from build123d import *

# Parameters (mm, degrees)
SKETCH1_R           = 2.75
BOSS_EXTRUDE1_DEPTH = 8
SKETCH5_R           = 2.25
BOSS_EXTRUDE2_DEPTH = 19
SKETCH6_R           = 6
BOSS_EXTRUDE4_DEPTH = 1.5
CUT_EXTRUDE1_DEPTH  = 1.5
CIRPATTERN1_COUNT   = 4
SKETCH11_R          = 1.4
BOSS_EXTRUDE5_DEPTH = 3
SKETCH12_R          = 2.2
BOSS_EXTRUDE6_DEPTH = 2.5


with BuildPart() as part:
    # Sketch1 → Boss-Extrude1 (new body)
    with BuildSketch(Plane.XY):
        with Locations((0, -0.147315355)):
            Circle(SKETCH1_R)
    extrude(amount=BOSS_EXTRUDE1_DEPTH)

    # Sketch4 → Revolve2 (revolve)
    with BuildSketch(Plane(origin=(0, 0, 0), x_dir=(1, 0, 0), z_dir=(0, 1, 0)), mode=Mode.PRIVATE) as revolve2_sk:
        Polygon((0, 0), (0, 2), (-2, 0), align=None)
    revolve(revolve2_sk.sketch.rotate(Axis((0, 0, 0), (0, 0, -1)), 180), axis=Axis((0, 0, 0), (0, 0, -1)))

    # Sketch5 → Boss-Extrude2 (add)
    with BuildSketch(Plane.XY.offset(8)):
        Circle(SKETCH5_R)
    extrude(amount=BOSS_EXTRUDE2_DEPTH)

    # Sketch6 → Boss-Extrude4 (add)
    with BuildSketch(Plane.XY.offset(8)):
        Circle(SKETCH6_R)
    extrude(amount=BOSS_EXTRUDE4_DEPTH)

    # Sketch7 → Cut-Extrude1 (cut)
    with BuildSketch(Plane(origin=(0, 0, 8), x_dir=(-1, 0, 0), z_dir=(0, 0, -1))):
        with BuildLine():
            ThreePointArc((0.5, -4.974937186), (3.535533906, -3.535533906), (4.974937186, -0.5))
            Line((4.974937186, -0.5), (2.727290513, -0.5))
            ThreePointArc((2.727290513, -0.5), (1.996550566, -2.038422395), (0.5, -2.851478812))
            Line((0.5, -2.851478812), (0.5, -4.974937186))
        make_face()
    cut_extrude1 = extrude(amount=-CUT_EXTRUDE1_DEPTH, mode=Mode.SUBTRACT)

    # CirPattern1: Cut-Extrude1 ×4 about axis
    cirpattern1_axis = Axis((0, 0, 0), (0, 0, 1))
    for i in range(1, CIRPATTERN1_COUNT):
        add(cut_extrude1.rotate(cirpattern1_axis, i * 360 / CIRPATTERN1_COUNT), mode=Mode.SUBTRACT)

    # Sketch10 → Revolve3 (revolve)
    with BuildSketch(Plane(origin=(0, 0, 0), x_dir=(0, 0, -1), z_dir=(1, 0, 0))):
        with BuildLine():
            Line((-27, 0), (-29, 0))
            Line((-29, 0), (-29, 1.4))
            add(Edge.make_bspline(
                [(-29, 1.4), (-28.086565691, 2.25), (-27, 2.25)],
                knots=[0, 0, 0, 1, 1, 1], degree=2))
            Line((-27, 2.25), (-27, 0))
        make_face()
    revolve(axis=Axis((0, 0, 27), (0, 0, 1)))

    # Sketch11 → Boss-Extrude5 (add)
    with BuildSketch(Plane.XY.offset(29)):
        Circle(SKETCH11_R)
    extrude(amount=BOSS_EXTRUDE5_DEPTH)

    # Sketch12 → Boss-Extrude6 (add)
    with BuildSketch(Plane.XY.offset(32)):
        Circle(SKETCH12_R)
    extrude(amount=BOSS_EXTRUDE6_DEPTH)


solid = part.part
Read the model definition and answer for the solid it produces. Units are mm, in the model's axes. A direction names the side the tool comes from. Give positions to 0.01 mm unless a question says otherwise; leave off trailing zeros. Write each loop counter-clockwise with the first axis right and the second up, starting at its lowest first coordinate (ties: lowest second). Pieces come first, ordered by that corner, then holes. Notation, with made-up numbers: (20.25, 1.5) - (34.25, 1.5) arc R33 ccw to (34.25, 33.5) - close; hole circle Ø11 at (15.5, 0.5). An arc over 180 degrees is marked (long way). Answer in a Markdown table with one row per item. Add a question column.
Item 1: Determine the mould class of faces 5 (the face through (0, 1, -1)), 6 (the face through (-0.5, -4, 9)), 7 (the face through (0, 3, 8)) for opening direction X: pulls with the +X half, pulls with the -X half, needs draft (parallel to the pull), parting line crosses it, or undercut.
Item 2: Section B-B, the plane z = 16 is taken. Write down the section's boundary in (x, y), and give its area (3 significant figures).
Item 3: Flat-ended cylindrical pins translate along their axes: P1, Ø1.6, axis at x = -4, z = 8.5, coming from the +Y side; P2, Ø1, axis at x = 0.5, y = -2.5, coming from the -Z side; P3, Ø0.8, axis at y = 4.5, z = 8.5, coming from the +X side; P4, Ø1, axis at x = 3, z = 28, coming from the +Y side. Find the tip coordinate at first contact, or state that the pin passes through.
Item 4: Section A-A, the plane x = -4 is taken. Write down the section's boundary in (y, z).
Item 5: Section C-C, the plane y = 1 is taken. Count the separate pieces of the cut face and the enclosed holes in it, and give its area (3 significant figures).
Item 6: A tool of negligible diameter and unlimited length cuts with its end or side. For faces 1 (the face through (-0.5, 4, 9)), 2 (the face through (1, -2, 0)), 3 (the face through (2.021, -2.013, 8.74)), 4 (the face through (0, 0, 34.5)), from which of +Z, -Z, +X, -X, +Y, -Y can it reach the whole face along a straight path? Write none if from no direction.
Item 7: Find the intervals of material crossed by L1, parallel to Y at x = -3.25, z = 8.5; L2, parallel to X at y = -0.5, z = 13.5; L3, parallel to Z at x = -1.5, y = 0.5, in increasing order.
Item 8: Section D-D, the plane z = 6 is taken. Write down the section's boundary in (x, y).
Recorded:
| question | item | result |
|---|---|---|
| 1 | face 5 | parting line crosses it |
| 1 | face 6 | undercut |
| 1 | face 7 | needs draft |
| 2 | outline | circle Ø4.5 at (0, 0) |
| 2 | area | 15.9 mm2 |
| 3 | P1 | stops at y = 5.08 |
| 3 | P2 | stops at z = 0 |
| 3 | P3 | stops at x = 4.38 |
| 3 | P4 | passes through |
| 4 | outline | (-4.47, 8) - (-3, 8) - (-3, 9.5) - (-4.47, 9.5) - close; (-0.5, 8) - (0.5, 8) - (0.5, 9.5) - (-0.5, 9.5) - close; (3, 8) - (4.47, 8) - (4.47, 9.5) - (3, 9.5) - close |
| 5 | separate pieces | 3 |
| 5 | enclosed holes | 0 |
| 5 | area | 146 mm2 |
| 6 | face 1 | +Z, -Z |
| 6 | face 2 | -Z |
| 6 | face 3 | +Z |
| 6 | face 4 | +Z, +X, -X, +Y, -Y |
| 7 | L1 | y = -5.04 to -3.8, -0.5 to 0.5, 3.8 to 5.04 |
| 7 | L2 | x = -2.19 to 2.19 |
| 7 | L3 | z = -0.42 to 28.79, 32 to 34.5 |
| 8 | outline | circle Ø5.5 at (0, -0.15) |
